from build123d import *

# Parameters (mm, degrees)
F_3_8_NPT_TAPPED_HOLE1_AT_2_COUNT = 2
F_3_8_NPT_TAPPED_HOLE1_AT_2_PITCH = 76.2
F_3_8_CLEARANCE_HOLE2_D           = 10.0838
CIRPATTERN1_COUNT                 = 10
F_1_8_NPT_TAPPED_HOLE2_AT_2_COUNT = 2
F_1_8_NPT_TAPPED_HOLE2_AT_2_PITCH = 38.1
SKETCH15_R                        = 3.175
CUT_EXTRUDE1_DEPTH                = 12.7


with BuildPart() as part:
    # Sketch1 → Revolve1 (revolve)
    with BuildSketch(Plane.XY):
        Polygon((0, 0), (-76.2, 0), (-76.2, -38.1), (-60.96, -38.1), (-60.96, -25.4), (-57.563361296, -25.4), (-57.563361296, -22.865513246), (-52.667748855, -22.865513246), (-52.667748855, -25.4), (-32.163982831, -25.4), (-30.364664072, -25.4), (-28.575, -25.4), (-28.575, -20.32), (-27.359482971, -20.32), (-27.359482971, -18.0238967), (-24.714766805, -18.0238967), (-24.714766805, -20.32), (-22.225, -20.32), (0, -15.85722), align=None)
    revolve(axis=Axis((0, 0, 0), (0, -1, 0)))

    # Sketch3 → 1/2 NPT Tapped Hole1 (revolve, cut)
    with BuildSketch(Plane(origin=(0, 0, 0), x_dir=(0, 0, 1), z_dir=(1, 0, 0))):
        Polygon((0, 0), (0, 38.1), (8.9281, 38.1), (8.9281, 13.462), (10.261665792, 13.462), (10.6647361, 0), align=None)
    revolve(axis=Axis((0, 6.35, 0), (0, -1, 0)), mode=Mode.SUBTRACT)

    # Sketch5 → 3/8 NPT Tapped Hole1 (revolve, cut)
    with BuildSketch(Plane(origin=(-38.1, 0, 0), x_dir=(0, 0, 1), z_dir=(1, 0, 0))):
        Polygon((0, 0), (0, 38.1), (7.1374, 38.1), (7.1374, 10.414), (8.263205494, 10.414), (8.5750146, 0), align=None)
    f_3_8_npt_tapped_hole1 = revolve(axis=Axis((-38.1, 6.35, 0), (0, -1, 0)), mode=Mode.SUBTRACT)

    # 3/8 NPT Tapped Hole1 at 2: 3/8 NPT Tapped Hole1 ×2
    with Locations(*[(i * F_3_8_NPT_TAPPED_HOLE1_AT_2_PITCH, 0, 0) for i in range(1, F_3_8_NPT_TAPPED_HOLE1_AT_2_COUNT)]):
        add(f_3_8_npt_tapped_hole1, mode=Mode.SUBTRACT)

    # 3/8 Clearance Hole2 (through all)
    with Locations(Plane(origin=(67.31, 0, 0), x_dir=(1, 0, 0), z_dir=(0, 1, 0))):
        with Locations((0, 0)):
            f_3_8_clearance_hole2 = Hole(F_3_8_CLEARANCE_HOLE2_D / 2)

    # CirPattern1: 3/8 Clearance Hole2 ×10 about axis
    cirpattern1_axis = Axis((0, 0, 0), (0, 1, 0))
    for i in range(1, CIRPATTERN1_COUNT):
        add(f_3_8_clearance_hole2.rotate(cirpattern1_axis, i * 360 / CIRPATTERN1_COUNT), mode=Mode.SUBTRACT)

    # Sketch7 → 1/8 NPT Tapped Hole2 (revolve, cut)
    with BuildSketch(Plane(origin=(-19.05, 0, -33.02), x_dir=(0, 0, 1), z_dir=(1, 0, 0))):
        Polygon((0, 0), (0, 38.1), (4.2164, 38.1), (4.2164, 6.858), (4.556413846, 6.858), (4.7427388, 0.635), (5.3777388, 0), align=None)
    f_1_8_npt_tapped_hole2 = revolve(axis=Axis((-19.05, 6.35, -33.02), (0, -1, 0)), mode=Mode.SUBTRACT)

    # 1/8 NPT Tapped Hole2 at 2: 1/8 NPT Tapped Hole2 ×2
    with Locations(*[(i * F_1_8_NPT_TAPPED_HOLE2_AT_2_PITCH, 0, 0) for i in range(1, F_1_8_NPT_TAPPED_HOLE2_AT_2_COUNT)]):
        add(f_1_8_npt_tapped_hole2, mode=Mode.SUBTRACT)

    # Sketch15 → Cut-Extrude1 (cut, symmetric)
    with BuildSketch(Plane(origin=(0, -0.843551224, -0.843551224), x_dir=(0, 0.707106781186549, -0.7071067811865461), z_dir=(0, -0.7071067811865461, -0.707106781186549))):
        with Locations((-25.322961582, 0)):
            Circle(SKETCH15_R)
    extrude(amount=CUT_EXTRUDE1_DEPTH, both=True, mode=Mode.SUBTRACT)

    # Sketch12 → 1/4 NPT Tapped Hole1 (revolve, cut)
    with BuildSketch(Plane(origin=(0, 0, 26.67), x_dir=(0, 0, 1), z_dir=(1, 0, 0))):
        Polygon((0, 0), (0, 16.51), (5.5626, 13.167652721), (5.5626, 9.906), (5.943685794, 9.906), (6.2402847, 0), align=None)
    revolve(axis=Axis((0, 6.35, 26.67), (0, -1, 0)), mode=Mode.SUBTRACT)


solid = part.part
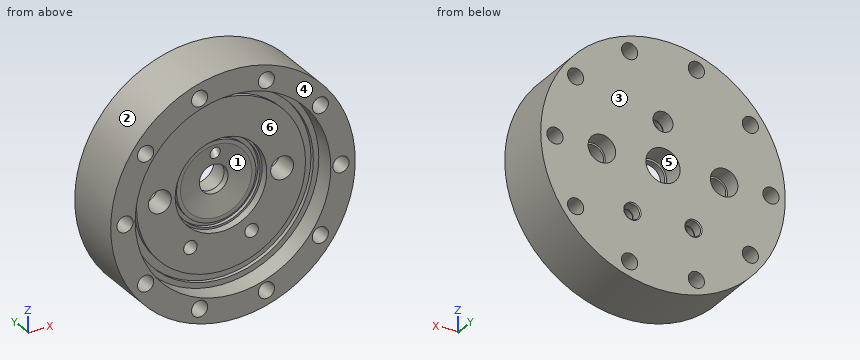
Build history of the part. All positions in model axes, mm. Face numbers are marked on the shaded views. A direction names the side the tool comes from. Give positions to 0.01 mm unless a question says otherwise; leave off trailing zeros. Order: outer loops, then holes, each group sorted by start corner. A loop starts at its lowest first (then second) coordinate and runs counter-clockwise, first axis right, second up. Notation, with made-up numbers: M 57,17 L 112,17 A24 cw 112,54 Z; hole C 49,-23 d3. An arc over 180 degrees is marked long. Use one line per item in the form item = value.
1) Tool access for the marked faces 4, 5 and 6: list every direction of +Z, -Z, +X, -X, +Y, -Y with a clear straight run to the whole face (end or side of a thin tool).
Calculated:
face_4 = +Z, -Z, +X, -X, -Y
face_5 = +Y
face_6 = -Y
2) Saw through at A-A (x = 67.31). Give the cut face in (y, z), plus the area to 3 significant figures.
Calculated:
outline = M -38.1,-35.72 L 0,-35.72 L 0,-5.04 L -38.1,-5.04 Z; M -38.1,5.04 L 0,5.04 L 0,35.72 L -38.1,35.72 Z
area = 2,340 mm2
3) Two-plate mould, pull along Z, no slides. Class the marked faces 1, 2 and 3: released by +Z, released by -Z, zero draft, split by the parting line, or undercut.
Calculated:
face_1 = undercut
face_2 = split by the parting line
face_3 = zero draft
4) Drop flat-ended pins along their axis: pin 1 (4 mm diameter, centred on x = -40.5, z = -11.5, fed in from -Y); pin 2 (10 mm diameter, centred on x = -40, y = -22.5, fed in from +Z); pin 3 (5 mm diameter, centred on y = -10.5, z = -3, fed in from -X). Give the stop position or say it passes through.
Calculated:
pin_1 = -25.4
pin_2 = 67.69
pin_3 = -76.2
5) Saw through at D-D (x = -38.1). Give the cut face in (y, z).
Calculated:
outline = M -38.1,-65.99 L 0,-65.99 L 0,-8.58 L -10.41,-8.26 L -10.41,-7.14 L -25.4,-7.14 L -25.4,-36.36 L -22.87,-36.36 L -22.87,-43.15 L -25.4,-43.15 L -25.4,-47.59 L -38.1,-47.59 Z; M -38.1,47.59 L -25.4,47.59 L -25.4,43.15 L -22.87,43.15 L -22.87,36.36 L -25.4,36.36 L -25.4,7.14 L -10.41,7.14 L -10.41,8.26 L 0,8.58 L 0,65.99 L -38.1,65.99 Z
6) Probe probe 1 along Z at (x, y) = (0, -24.65) (3 decimals); probe 2 along Z at (x, y) = (23, -33); probe 3 along X at (y, z) = (-14, -29.5). List the from-to ranges inside material, lowest first.
Calculated:
probe_1 = -76.2 to -57.563, -52.668 to -28.575, 28.575 to 52.668, 57.563 to 76.2
probe_2 = -72.65 to -68.55, -59.48 to -56.45, 56.45 to 59.48, 68.55 to 72.65
probe_3 = -70.26 to -21.37, -16.73 to 16.73, 21.37 to 70.26
7) Saw through at B-B (y = -32). State how many separate pieces and enclosed holes the cut face has, plus the area to 3 significant figures.
Calculated:
separate_pieces = 1
enclosed_holes = 11
area = 5,770 mm2
